Design review of the part built by this model. Coordinates are the model's own, in mm. A direction names the side the tool comes from. Coordinates: 2 decimals unless noted, no trailing zeros. Order: outer loops, then holes, each group sorted by start corner. A loop starts at its lowest first (then second) coordinate and runs counter-clockwise, first axis right, second up. Notation, with made-up numbers: (69.25, 83) -> (106.25, 83) arc R32 cw to (106.25, 114) -> close; hole circle Ø2 at (81.5, 40). An arc over 180 degrees is marked (long way). Write item = value, one per line.
```python
from build123d import *

# Parameters (mm, degrees)
BOSS_EXTRUDE1_DEPTH = 30
FILLET1_R           = 10
SKETCH4_R           = 4
CUT_EXTRUDE1_DEPTH  = 3
SKETCH5_R           = 1.5
CUT_EXTRUDE2_DEPTH  = 3


with BuildPart() as part:
    # Sketch1 → Boss-Extrude1 (new body)
    with BuildSketch(Plane.XY):
        Polygon((0, 0), (0, 40), (-30, 40), (-30, 0), (-32, 0), (-32, 42), (2, 42), (2, 0), align=None)
    extrude(amount=BOSS_EXTRUDE1_DEPTH)

    # Fillet1
    fillet1_edges = [part.edges().sort_by_distance(p)[0] for p in [
        (1, 0, 0),
        (-31, 0, 30),
        (1, 0, 30),
        (-31, 0, 0),
    ]]
    fillet(fillet1_edges, radius=FILLET1_R)

    # Sketch4 → Cut-Extrude1 (cut)
    with BuildSketch(Plane.ZY.offset(32)):
        with Locations(Location((15.066442129, 8.440123405, 0), (0, 0, 270))):
            Circle(SKETCH4_R)
    extrude(amount=-CUT_EXTRUDE1_DEPTH, mode=Mode.SUBTRACT)

    # Sketch5 → Cut-Extrude2 (cut)
    with BuildSketch(Plane(origin=(2, 0, 0), x_dir=(0, 0, -1), z_dir=(1, 0, 0))):
        with Locations((-15.066442129, 8.440123405)):
            Circle(SKETCH5_R)
    extrude(amount=-CUT_EXTRUDE2_DEPTH, mode=Mode.SUBTRACT)


solid = part.part
```
(1) We need section C-C (x = -0.5). Write out the cut boundary in (y, z), and give its area (3 significant figures).
Report:
outline = (40, 0) -> (42, 0) -> (42, 30) -> (40, 30) -> close
area = 60.0 mm²
(2) We need section A-A (y = 21.5). Write out the cut boundary in (x, z).
Report:
outline = (-32, 0) -> (-30, 0) -> (-30, 30) -> (-32, 30) -> close; (0, 0) -> (2, 0) -> (2, 30) -> (0, 30) -> close
(3) We need section D-D (z = 26.5). Write out the cut boundary in (x, y).
Report:
outline = (-32, 2.4) -> (-30, 2.4) -> (-30, 40) -> (0, 40) -> (0, 2.4) -> (2, 2.4) -> (2, 42) -> (-32, 42) -> close
(4) We need section B-B (z = 2.75). Write out the cut boundary in (x, y).
Report:
outline = (-32, 3.11) -> (-30, 3.11) -> (-30, 40) -> (0, 40) -> (0, 3.11) -> (2, 3.11) -> (2, 42) -> (-32, 42) -> close
(5) The part is to be moulded in two halves that separate along Z. For faces 1 (the cylindrical face through (1.01, 7.87, 13.68)), 2 (the cylindrical face through (0.99, 2.85, 26.99)), 3 (the flat face through (0, 20, 15)), say which applies: released by +Z, released by -Z, zero draft, split by the parting line, or undercut.
Report:
face_1 = undercut
face_2 = released by +Z
face_3 = zero draft
(6) Insertion check: pin 1 (7 mm diameter, centred on y = 8.44, z = 15.07, fed in from -X); pin 2 (15 mm diameter, centred on x = -11.5, z = 22, fed in from -Y). Each pin has a flat end and moves straight along its axis. Give the tip position at first contact, or say it passes through.
Report:
pin_1 = 0
pin_2 = 40
(7) For L1, parallel to X at y = 24.5, z = 6.25; L2, parallel to Y at x = -17.5, z = 20.25; L3, parallel to X at y = 7, z = 13, list the stretches that pass through material, from the lowest coordinate up.
Report:
L1 = -32 to -30, 0 to 2
L2 = 40 to 42
L3 = 0 to 2
(8) For faces 4 (the cylindrical face through (-31.01, 2.85, 26.99)), 5 (the flat face through (-30, 20, 15)), 6 (the cylindrical face through (-31.014, 8.961, 19.032)), list the 3-axis set-ups (+Z, -Z, +X, -X, +Y, -Y) from which the entire face can be reached by the end or side of a thin tool; tool diameter is ignored.
Report:
face_4 = +Z, +X, -X, -Y
face_5 = +Z, -Z, -Y
face_6 = -X
